Check sheet for the modelled part. Datum: model origin and axes. Units: mm. Face numbers are marked on the shaded views. A direction names the side the tool comes from. Give positions to 0.01 mm unless a question says otherwise; leave off trailing zeros. Write each loop counter-clockwise with the first axis right and the second up, starting at its lowest first coordinate (ties: lowest second). Pieces come first, ordered by that corner, then holes. Notation, with made-up numbers: M 19.5,-30 L 77.5,-30 A24 cw 77.5,4 Z; hole C 40.25,12 d5. An arc over 180 degrees is marked long. Write item = value, one per line. Start each with the question number.
1) Gauge pin test, flat ends, axial feed: pin 1 (1.5 mm diameter, centred on x = 1.5, y = -2, fed in from -Z); pin 2 (0.8 mm diameter, centred on x = 0, y = 0.5, fed in from -Z). Record the tip position at first contact, or that the pin passes through.
2) Scan lines: L1, parallel to Z at x = -0.55, y = -1.55; L2, parallel to Z at x = -0.4, y = 1.05; L3, parallel to X at y = -0.3, z = 1.25. Record each from-to range of solid material in increasing order.
3) Sectioned sample at A-A, the plane x = 0. Record the cut outline in (y, z).
4) Sectioned sample at B-B, the plane y = -0.6. Record the cut outline in (x, z), then the cut area to 3 significant figures.
5) Sectioned sample at D-D, the plane x = 2.2. Record the cut outline in (y, z).
6) Sectioned sample at C-C, the plane z = 18.75. Record the cut outline in (x, y), then the cut area to 3 significant figures.
7) Set-up check for the marked faces 1 and 2: record each of +Z, -Z, +X, -X, +Y, -Y from which the full face is reachable in a straight line by a thin tool's end or side.
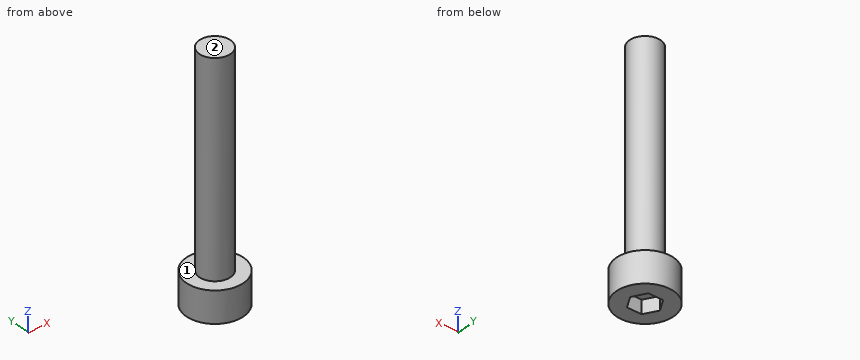
Autodesk Inventor part; units mm, degrees
ref_plane "YZ Plane" through (0, 0, 0) normal (1, 0, 0) x (0, 1, 0)
ref_plane "XZ Plane" through (0, 0, 0) normal (0, 1, 0) x (-1, 0, 0)
ref_plane "XY Plane" through (0, 0, 0) normal (0, 0, 1) x (1, 0, 0)
sketch "Sketch1" plane through (0, 0, 0) normal (0, 1, 0) x (-1, 0, 0)
  line L0 (0, 0) -> (-2.75, 0)
  line L1 (-2.75, 0) -> (-2.75, 3)
  line L2 (-2.75, 3) -> (-1.5, 3)
  line L3 (-1.5, 3) -> (-1.5, 23)
  line L4 (-1.5, 23) -> (0, 23)
  line L5 (0, 23) -> (0, 0)
  dimension "ScrewLength" = 20
  dimension "Diameter" = 5.5
  dimension "Metric" = 3
  dimension "HeadLength" = 3
revolve "Revolution1" add sketch "Sketch1" angle 360 about axis through (0, 0, 23) along (0, 0, -1)
thread "Thread1"
sketch "Sketch2" plane through (0, 0, 0) normal (0, 0, -1) x (-1, 0, 0)
  line L0 (0.7217, 1.25) -> (1.4434, 0)
  line L1 (1.4434, 0) -> (0.7217, -1.25)
  line L2 (0.7217, -1.25) -> (-0.7217, -1.25)
  line L3 (-0.7217, -1.25) -> (-1.4434, 0)
  line L4 (-1.4434, 0) -> (-0.7217, 1.25)
  line L5 (-0.7217, 1.25) -> (0.7217, 1.25)
  point P0 (0, 0)
  point P1 (0, 0)
  dimension "WidthAcrossFlat" = 2.5
extrude "Extrusion1" cut sketch "Sketch2" against normal blind 1.3
properties part number "UC-0320" material "Stainless Steel AISI 304"
Data:
q1.pin_1 = 0
q1.pin_2 = 1.3
q2.L1 = 0 to 3
q2.L2 = 1.3 to 23
q2.L3 = -2.73 to -1.27, 1.27 to 2.73
q3.outline = M -2.75,0 L -1.25,0 L -1.25,1.3 L 1.25,1.3 L 1.25,0 L 2.75,0 L 2.75,3 L 1.5,3 L 1.5,23 L -1.5,23 L -1.5,3 L -2.75,3 Z
q4.outline = M -2.68,0 L -1.1,0 L -1.1,1.3 L 1.1,1.3 L 1.1,0 L 2.68,0 L 2.68,3 L 1.37,3 L 1.37,23 L -1.37,23 L -1.37,3 L -2.68,3 Z
q4.area = 68.2 mm2
q5.outline = M -1.65,0 L 1.65,0 L 1.65,3 L -1.65,3 Z
q6.outline = C 0,0 d3
q6.area = 7.07 mm2
q7.face_1 = +Z
q7.face_2 = +Z, +X, -X, +Y, -Y
